Check sheet for the modelled part. Datum: model origin and axes. Units: mm. Round coordinates to 2 decimals unless told otherwise and drop trailing zeros. Order: outer loops, then holes, each group sorted by start corner. A loop starts at its lowest first (then second) coordinate and runs counter-clockwise, first axis right, second up. Notation, with made-up numbers: (8, 33) -> (45, 33) arc R29 cw to (45, 71) -> close; hole circle Ø7 at (9, -27). An arc over 180 degrees is marked (long way). Answer in a Markdown table with one row per item.
from build123d import *

# Parameters (mm, degrees)
SKETCH_1_R      = 2
SKETCH_1_R_2    = 2.05
SKETCH_1_R_3    = 5
EXTRUDE_1_DEPTH = 2


with BuildPart() as part:
    # 草图1 → 凸台-拉伸1 (new body)
    with BuildSketch(Plane(origin=(0, 0, 0), x_dir=(1, 0, 0), z_dir=(0, 1, 0))):
        Polygon((-31.5, -48), (-21.75, -48), (-21.75, -51), (-13.75, -51), (-13.75, -48), (13.75, -48), (13.75, -51), (21.75, -51), (21.75, -48), (31.5, -48), (31.5, -45.5), (30, -45.5), (30, -42.9), (31.5, -42.9), (31.5, -39.9), (34.5, -39.9), (34.5, -42.9), (36, -42.9), (36, -45.5), (34.5, -45.5), (34.5, -48), (35.5, -48), (47.5, -48), (48, -48), (48, -35.5), (48, -34.5), (45.5, -34.5), (45.5, -36), (42.9, -36), (42.9, -34.5), (39.9, -34.5), (39.9, -31.5), (42.9, -31.5), (42.9, -30), (45.5, -30), (45.5, -31.5), (48, -31.5), (48, -21.75), (51, -21.75), (51, -13.75), (48, -13.75), (48, 13.75), (51, 13.75), (51, 21.75), (48, 21.75), (48, 31.5), (45.5, 31.5), (45.5, 30), (42.9, 30), (42.9, 31.5), (39.9, 31.5), (39.9, 34.5), (42.9, 34.5), (42.9, 36), (45.5, 36), (45.5, 34.5), (48, 34.5), (48, 46.5), (48, 48), (35.5, 48), (34.5, 48), (34.5, 45.5), (36, 45.5), (36, 42.9), (34.5, 42.9), (34.5, 39.9), (31.5, 39.9), (31.5, 42.9), (30, 42.9), (30, 45.5), (31.5, 45.5), (31.5, 48), (21.75, 48), (21.75, 51), (13.75, 51), (13.75, 48), (-13.75, 48), (-13.75, 51), (-21.75, 51), (-21.75, 48), (-31.5, 48), (-31.5, 45.5), (-30, 45.5), (-30, 42.9), (-31.5, 42.9), (-31.5, 39.9), (-34.5, 39.9), (-34.5, 42.9), (-36, 42.9), (-36, 45.5), (-34.5, 45.5), (-34.5, 48), (-42.9, 48), (-48, 48), (-48, 47), (-48, 34.5), (-45.5, 34.5), (-45.5, 36), (-42.9, 36), (-42.9, 34.5), (-39.9, 34.5), (-39.9, 31.5), (-42.9, 31.5), (-42.9, 30), (-45.5, 30), (-45.5, 31.5), (-48, 31.5), (-48, 21.75), (-51, 21.75), (-51, 13.75), (-48, 13.75), (-48, -13.75), (-51, -13.75), (-51, -21.75), (-48, -21.75), (-48, -31.5), (-45.5, -31.5), (-45.5, -30), (-42.9, -30), (-42.9, -31.5), (-39.9, -31.5), (-39.9, -34.5), (-42.9, -34.5), (-42.9, -36), (-45.5, -36), (-45.5, -34.5), (-48, -34.5), (-48, -35.5), (-48, -48), (-47, -48), (-34.5, -48), (-34.5, -45.5), (-36, -45.5), (-36, -42.9), (-34.5, -42.9), (-34.5, -39.9), (-31.5, -39.9), (-31.5, -42.9), (-30, -42.9), (-30, -45.5), (-31.5, -45.5), align=None)
        with Locations(Location((0, -15, 0), (0, 0, 270))):
            Circle(SKETCH_1_R, mode=Mode.SUBTRACT)
        with Locations(Location((-12.990381057, -7.5, 0), (0, 0, 270))):
            Circle(SKETCH_1_R, mode=Mode.SUBTRACT)
        with Locations(Location((-12.990381057, 7.5, 0), (0, 0, 270))):
            Circle(SKETCH_1_R, mode=Mode.SUBTRACT)
        with Locations(Location((0, 15, 0), (0, 0, 270))):
            Circle(SKETCH_1_R, mode=Mode.SUBTRACT)
        with Locations(Location((12.990381057, 7.5, 0), (0, 0, 270))):
            Circle(SKETCH_1_R, mode=Mode.SUBTRACT)
        with Locations(Location((12.990381057, -7.5, 0), (0, 0, 270))):
            Circle(SKETCH_1_R, mode=Mode.SUBTRACT)
        with Locations(Location((-13.53, 0, 0), (0, 0, 270))):
            Circle(SKETCH_1_R_2, mode=Mode.SUBTRACT)
        with Locations(Location((6.765, 11.717323713, 0), (0, 0, 270))):
            Circle(SKETCH_1_R_2, mode=Mode.SUBTRACT)
        with Locations(Location((6.765, -11.717323713, 0), (0, 0, 270))):
            Circle(SKETCH_1_R_2, mode=Mode.SUBTRACT)
        with Locations(Location((0, 0, 0), (0, 0, 270))):
            Circle(SKETCH_1_R_3, mode=Mode.SUBTRACT)
    extrude(amount=EXTRUDE_1_DEPTH)


solid = part.part
Item 1: Cross-section at A-A (z = -41.5). Record the boundary of the cut face in (x, y).
Result sheet:
| item | result |
|---|---|
| outline | (-48, 0) -> (-34.5, 0) -> (-34.5, 2) -> (-48, 2) -> close; (-31.5, 0) -> (31.5, 0) -> (31.5, 2) -> (-31.5, 2) -> close; (34.5, 0) -> (48, 0) -> (48, 2) -> (34.5, 2) -> close |
Item 2: Cross-section at B-B (x = 0). Record the boundary of the cut face in (y, z).
Result sheet:
| item | result |
|---|---|
| outline | (0, -48) -> (2, -48) -> (2, -17) -> (0, -17) -> close; (0, -13) -> (2, -13) -> (2, -5) -> (0, -5) -> close; (0, 5) -> (2, 5) -> (2, 13) -> (0, 13) -> close; (0, 17) -> (2, 17) -> (2, 48) -> (0, 48) -> close |
Item 3: Depth check by flat-ended pin: P1, Ø0.8, axis at x = -35.5, y = 1, coming from the +Z side; P2, Ø1.2, axis at y = 0.5, z = -35, coming from the +X side; P3, Ø0.6, axis at x = 32.5, y = 1, coming from the +Z side. Enter the tip coordinate at first touch or a pass-through.
Result sheet:
| item | result |
|---|---|
| P1 | stops at z = 48 |
| P2 | stops at x = 48 |
| P3 | stops at z = 39.9 |
Item 4: Scan lines: line 1 (X direction, y = 1.45, z = -41); line 2 (X direction, y = 0.5, z = 0). Record each from-to range of solid material in increasing order. Write a range as [from, to].
Result sheet:
| item | result |
|---|---|
| line 1 | x = [-48, -34.5], [-31.5, 31.5], [34.5, 48] |
| line 2 | x = [-48, -15.58], [-11.48, -5], [5, 48] |
Item 5: Cross-section at D-D (z = -7.5). Record the boundary of the cut face in (x, y).
Result sheet:
| item | result |
|---|---|
| outline | (-48, 0) -> (-14.99, 0) -> (-14.99, 2) -> (-48, 2) -> close; (-10.99, 0) -> (10.99, 0) -> (10.99, 2) -> (-10.99, 2) -> close; (14.99, 0) -> (48, 0) -> (48, 2) -> (14.99, 2) -> close |
Item 6: Cross-section at C-C (z = 15). Record the boundary of the cut face in (x, y), and give its area (3 significant figures).
Result sheet:
| item | result |
|---|---|
| outline | (-51, 0) -> (-2, 0) -> (-2, 2) -> (-51, 2) -> close; (2, 0) -> (51, 0) -> (51, 2) -> (2, 2) -> close |
| area | 196 mm^2 |
Item 7: Mould release check, pull along Z, two halves, no side actions. Record for faces 1 (the cylindrical face through (-4.88, 0.99, -1.08)), 2 (the flat face through (-1, 2, -12)): pulls with the +Z half, pulls with the -Z half, needs draft (parallel to the pull), parting line crosses it, or undercut.
Result sheet:
| item | result |
|---|---|
| face 1 | undercut |
| face 2 | needs draft |
